Source: three-view drawing plus pictorial views. Frame: mm from the lowest corner of the part. Round coordinates to 2 decimals unless told otherwise and drop trailing zeros. Loops run counter-clockwise (first coordinate to the right, second up) from the corner with the lowest first, then second, coordinate; pieces in that order, holes last. Notation, with made-up numbers: (61, 88) -> (78, 88) arc R20 ccw to (78, 123) -> close; hole circle Ø5 at (14, 83). An arc over 180 degrees is marked (long way). Put each result on its own line as item: value. Start each with the question number.
1. Cut plane D-D (z = 179). Return the cut outline in (x, y) (3 decimals).
2. Cut plane B-B (x = 25). Return the cut outline in (y, z) (3 decimals).
3. Cut plane C-C (x = 40.5). Return the cut outline in (y, z) (3 decimals).
4. Material intervals for L1, parallel to X at y = 0.65, z = 142.5; L2, parallel to Z at x = 40.5, y = 2.95 (3 decimals); L3, parallel to Z at x = 40, y = 2.2, sorted ascending.
5. Contact query for a flat-ended pin moving along its axis: pin 1 (1 mm diameter, centred on y = 1.5, z = 169, fed in from +X). Output: stop coordinate, or through.
6. Cut plane A-A (y = 1.5). Return the cut outline in (x, z) (3 decimals).
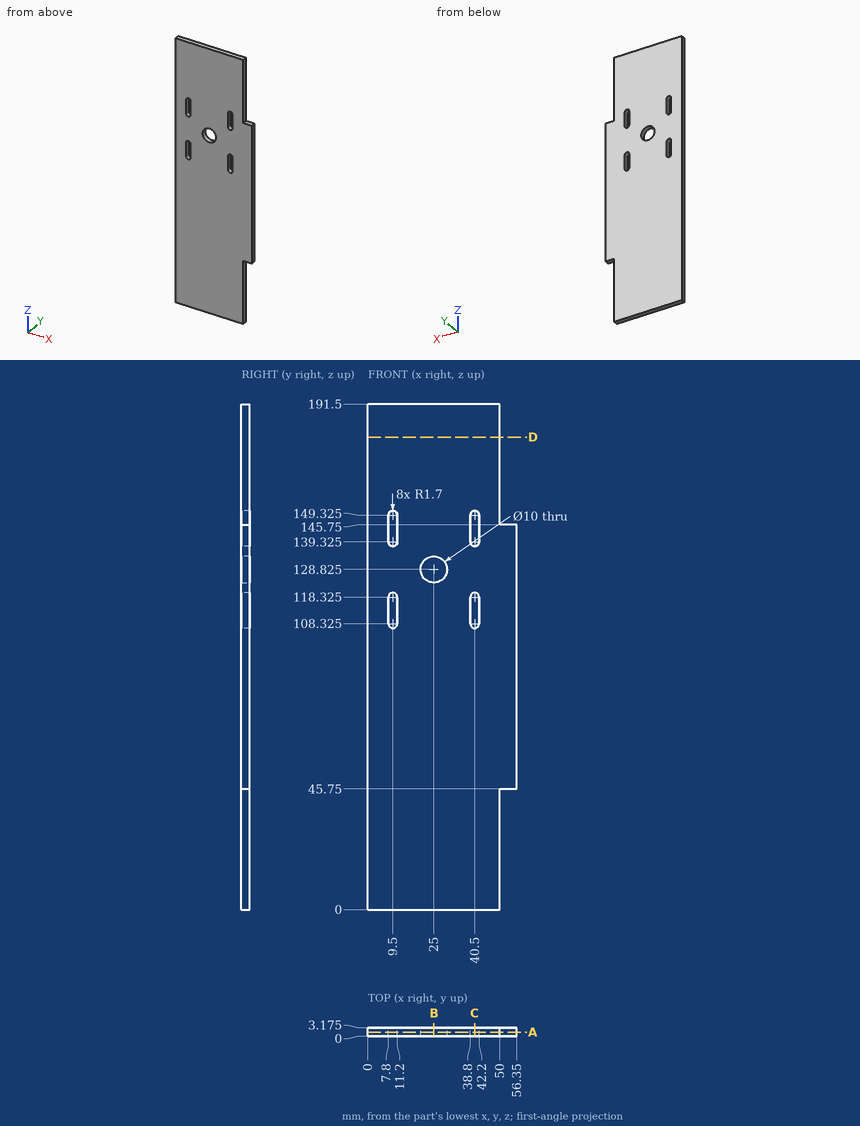
Solution:
1. outline: (0, 0) -> (50, 0) -> (50, 3.175) -> (0, 3.175) -> close
2. outline: (0, 0) -> (3.175, 0) -> (3.175, 123.825) -> (0, 123.825) -> close; (0, 133.825) -> (3.175, 133.825) -> (3.175, 191.5) -> (0, 191.5) -> close
3. outline: (0, 0) -> (3.175, 0) -> (3.175, 106.625) -> (0, 106.625) -> close; (0, 120.025) -> (3.175, 120.025) -> (3.175, 137.625) -> (0, 137.625) -> close; (0, 151.025) -> (3.175, 151.025) -> (3.175, 191.5) -> (0, 191.5) -> close
4. L1: x = 0 to 7.8, 11.2 to 38.8, 42.2 to 56.35
4. L2: z = 0 to 106.625, 120.025 to 137.625, 151.025 to 191.5
4. L3: z = 0 to 106.7, 119.95 to 137.7, 150.95 to 191.5
5. pin 1: stops at x = 50
6. outline: (0, 0) -> (50, 0) -> (50, 45.75) -> (56.35, 45.75) -> (56.35, 145.75) -> (50, 145.75) -> (50, 191.5) -> (0, 191.5) -> close; hole (7.8, 108.325) arc R1.7 ccw to (11.2, 108.325) -> (11.2, 118.325) arc R1.7 ccw to (7.8, 118.325) -> close; hole (7.8, 139.325) arc R1.7 ccw to (11.2, 139.325) -> (11.2, 149.325) arc R1.7 ccw to (7.8, 149.325) -> close; hole circle Ø10 at (25, 128.825); hole (38.8, 108.325) arc R1.7 ccw to (42.2, 108.325) -> (42.2, 118.325) arc R1.7 ccw to (38.8, 118.325) -> close; hole (38.8, 139.325) arc R1.7 ccw to (42.2, 139.325) -> (42.2, 149.325) arc R1.7 ccw to (38.8, 149.325) -> close
